Part model, mm, in its own coordinate system. A direction names the side the tool comes from. Round coordinates to 2 decimals unless told otherwise and drop trailing zeros. Order: outer loops, then holes, each group sorted by start corner. A loop starts at its lowest first (then second) coordinate and runs counter-clockwise, first axis right, second up. Notation, with made-up numbers: (36, 76) - (64, 76) arc R24 cw to (64, 92) - close; hole circle Ø6 at (11.25, -35). An arc over 180 degrees is marked (long way). Answer as a JSON object with one key per item and string values.
```python
from build123d import *

# Parameters (mm, degrees)
RESSALTO_EXTRUS_O1_DEPTH                             = 1000
CORTE_EXTRUS_O1_START                                = -1000
CORTE_EXTRUS_O1_DEPTH                                = 1000
CORTE_EXTRUS_O2_DEPTH                                = 1001.031261626
CORTE_EXTRUS_O3_DEPTH                                = 1001.031261626
CORTE_EXTRUS_O4_DEPTH                                = 1001.031261626
CORTE_EXTRUS_O5_DEPTH                                = 0.002166667
CORTE_EXTRUS_O6_DEPTH                                = 0.002166667
CORTE_EXTRUS_O7_DEPTH                                = 0.002166667
CORTE_EXTRUS_O8_DEPTH                                = 0.002166667
INCLINA_O1_ANGLE                                     = 45.1469538
ESBO_O10_W                                           = 0.450000001
ESBO_O10_H                                           = 1000
REBAIXO_PARA_PARAFUSO_DE_M_QUINA_DE_CABE_D           = 3.5
REBAIXO_PARA_PARAFUSO_DE_M_QUINA_DE_CABE_CBORE_D     = 6
REBAIXO_PARA_PARAFUSO_DE_M_QUINA_DE_CABE_CBORE_DEPTH = 3.50000002
CHANFRO1_SIZE                                        = 0.062563219
CHANFRO1_SIZE2                                       = 0.062205617
CHANFRO3_START                                       = -3.730761794
CHANFRO3_DEPTH                                       = 0.399013115
CHANFRO4_SIZE                                        = 0.4
FILETE1_R                                            = 0.130000023
SKETCH1_W                                            = 36.072768502
SKETCH1_H                                            = 858.120887339
SKETCH1_W_2                                          = 21.632087489
SKETCH1_H_2                                          = 62.411000867
CUT_EXTRUDE1_DEPTH                                   = 10


with BuildPart() as part:
    # Esboço1 → Ressalto-extrusão1 (new body)
    with BuildSketch(Plane.XZ):
        with BuildLine():
            Line((4.5, 5.4097155), (4.5, 6.01167813))
            Line((4.5, 6.01167813), (4.1, 6.50000002))
            Line((4.1, 6.50000002), (-4.1, 6.50000002))
            Line((-4.1, 6.50000002), (-4.5, 6.01167813))
            Line((-4.5, 6.01167813), (-4.5, 2e-08))
            Line((-4.5, 2e-08), (4.5, 2e-08))
            Line((4.5, 2e-08), (4.5, 3.50196265))
            ThreePointArc((4.5, 3.50196265), (4.477413879, 3.553810372), (4.43494978, 3.59116167))
            ThreePointArc((4.43494978, 3.59116167), (3.930462682, 4.43021964), (4.43494978, 5.26927761))
            ThreePointArc((4.43494978, 5.26927761), (4.490651601, 5.328761203), (4.5, 5.4097155))
        make_face()
    extrude(amount=-RESSALTO_EXTRUS_O1_DEPTH)

    # Esboço2 → Corte-extrusão1 (cut)
    with BuildSketch(Plane(origin=(0, 1000, 0), x_dir=(-1, 0, 0), z_dir=(0, 1, 0)).offset(CORTE_EXTRUS_O1_START)):
        with BuildLine():
            Line((-4.030498711, 4.00588336), (-3.673447948, 4.00588336))
            ThreePointArc((-3.673447948, 4.00588336), (-3.223447946, 4.455883362), (-3.673447948, 4.905883363))
            Line((-3.673447948, 4.905883363), (-3.953580008, 4.905883363))
            ThreePointArc((-3.953580008, 4.905883363), (-4.010719931, 4.899199784), (-4.065149208, 4.917830263))
            ThreePointArc((-4.065149208, 4.917830263), (-3.93114763, 4.466290066), (-4.030498711, 4.00588336))
        make_face()
    extrude(amount=CORTE_EXTRUS_O1_DEPTH, mode=Mode.SUBTRACT)

    # Esboço3 → Corte-extrusão2 (cut, through all)
    with BuildSketch(Plane(origin=(0, 1000, 0), x_dir=(-1, 0, 0), z_dir=(0, 1, 0))):
        with BuildLine():
            Line((4.5, 4.03150278), (4.5, 4.88017535))
            Line((4.5, 4.88017535), (3.66946318, 4.88017535))
            ThreePointArc((3.66946318, 4.88017535), (3.969667593, 4.455839065), (3.66946318, 4.03150278))
            Line((3.66946318, 4.03150278), (4.5, 4.03150278))
        make_face()
    extrude(amount=-CORTE_EXTRUS_O2_DEPTH, mode=Mode.SUBTRACT)

    # Esboço4 → Corte-extrusão3 (cut, through all)
    with BuildSketch(Plane(origin=(0, 1000, 0), x_dir=(-1, 0, 0), z_dir=(0, 1, 0))):
        with BuildLine():
            Line((4.026513974, 4.88017535), (4.5, 4.88017535))
            Line((4.5, 4.88017535), (4.5, 5.328056964))
            ThreePointArc((4.5, 5.328056964), (4.223646078, 5.145991535), (4.026513974, 4.88017535))
        make_face()
    extrude(amount=-CORTE_EXTRUS_O3_DEPTH, mode=Mode.SUBTRACT)

    # Esboço5 → Corte-extrusão4 (cut, through all)
    with BuildSketch(Plane(origin=(0, 1000, 0), x_dir=(-1, 0, 0), z_dir=(0, 1, 0))):
        with BuildLine():
            Line((4.5, 3.583620931), (4.5, 4.03150278))
            Line((4.5, 4.03150278), (4.026513856, 4.03150278))
            ThreePointArc((4.026513856, 4.03150278), (4.223645982, 3.76568645), (4.5, 3.583620931))
        make_face()
    extrude(amount=-CORTE_EXTRUS_O4_DEPTH, mode=Mode.SUBTRACT)

    # Esboço6 → Corte-extrusão5 (cut)
    with BuildSketch(Plane(origin=(0, 1000, 0), x_dir=(-1, 0, 0), z_dir=(0, 1, 0))):
        Polygon((0.891369267, 3.403698133), (0.714701433, 3.168235633), (0.2187042, 2.61105), (1.0945792, 2.61105), (1.0945792, 2.695983333), (0.398689633, 2.695983333), (0.794326433, 3.149466667), (0.9743123, 3.3891), (1.067110588, 3.573407857), (0.95413722, 3.802321701), (0.7876908, 3.88505), (0.54301, 3.88505), (0.375434678, 3.803592619), (0.295011167, 3.6384023), (0.295011167, 3.562), (0.3812718, 3.562), (0.3812718, 3.631766667), (0.437672733, 3.743620833), (0.549645633, 3.800116667), (0.7802262, 3.800116667), (0.893028067, 3.743810633), (0.976240026, 3.576039029), align=None)
    extrude(amount=-CORTE_EXTRUS_O5_DEPTH, mode=Mode.SUBTRACT)

    # Esboço7 → Corte-extrusão6 (cut)
    with BuildSketch(Plane.XZ):
        Polygon((-0.214632167, 3.88505), (-0.953983333, 3.88505), (-0.953983333, 2.61105), (-0.214632167, 2.61105), (-0.214632167, 2.695983333), (-0.86905, 2.695983333), (-0.86905, 3.205583333), (-0.5123963, 3.205583333), (-0.5123963, 3.290516667), (-0.86905, 3.290516667), (-0.86905, 3.800116667), (-0.214632167, 3.800116667), align=None)
    extrude(amount=-CORTE_EXTRUS_O6_DEPTH, mode=Mode.SUBTRACT)

    # Esboço8 → Corte-extrusão7 (cut)
    with BuildSketch(Plane(origin=(0, 1000, 0), x_dir=(-1, 0, 0), z_dir=(0, 1, 0))):
        Polygon((-0.214632167, 3.88505), (-0.953983333, 3.88505), (-0.953983333, 2.61105), (-0.214632167, 2.61105), (-0.214632167, 2.695983333), (-0.86905, 2.695983333), (-0.86905, 3.205583333), (-0.5123963, 3.205583333), (-0.5123963, 3.290516667), (-0.86905, 3.290516667), (-0.86905, 3.800116667), (-0.214632167, 3.800116667), align=None)
    extrude(amount=-CORTE_EXTRUS_O7_DEPTH, mode=Mode.SUBTRACT)

    # Esboço9 → Corte-extrusão8 (cut)
    with BuildSketch(Plane.XZ):
        Polygon((0.510057167, 3.620830633), (0.6071, 3.718655633), (0.6071, 2.609403333), (0.692033333, 2.609403333), (0.692033333, 3.883403333), (0.6741176, 3.883403333), (0.6741176, 3.795069794), (0.3690544, 3.640736667), (0.3690544, 3.551253333), align=None)
    extrude(amount=-CORTE_EXTRUS_O8_DEPTH, mode=Mode.SUBTRACT)

    # Inclinação1
    inclina_o1_faces = [part.faces().sort_by_distance(p)[0] for p in [
        (0.6741176, 0.001083333, 3.839236564),
    ]]
    draft(inclina_o1_faces, Plane(origin=(0.692033333, 0.002166667, 3.883403333), x_dir=(-1, 0, 0), z_dir=(0, 0, -1)), INCLINA_O1_ANGLE)

    # Esboço10 → Corte-Revolução1 (revolve, cut)
    with BuildSketch(Plane.XY.offset(4.455839065)):
        with Locations((-3.294667591, 500)):
            Rectangle(ESBO_O10_W, ESBO_O10_H)
    revolve(axis=Axis((-3.519667591, 1000, 4.455839065), (0, -1, 0)), mode=Mode.SUBTRACT)

    # Rebaixo para parafuso de máquina de cabeça sextavada de M31 (through all)
    with Locations(Plane.XY.offset(6.50000002)):
        with Locations((0, 990), (0, 970), (0, 950), (0, 930), (0, 910), (0, 890), (0, 870), (0, 850), (0, 830), (0, 810), (0, 790), (0, 770), (0, 750), (0, 730), (0, 710), (0, 690), (0, 670), (0, 650), (0, 630), (0, 610), (0, 590), (0, 570), (0, 550), (0, 530), (0, 510), (0, 490), (0, 470), (0, 450), (0, 430), (0, 410), (0, 390), (0, 370), (0, 350), (0, 330), (0, 310), (0, 290), (0, 270), (0, 250), (0, 230), (0, 210), (0, 190), (0, 170), (0, 150), (0, 130), (0, 110), (0, 90), (0, 70), (0, 50), (0, 30), (0, 10)):
            CounterBoreHole(REBAIXO_PARA_PARAFUSO_DE_M_QUINA_DE_CABE_D / 2, REBAIXO_PARA_PARAFUSO_DE_M_QUINA_DE_CABE_CBORE_D / 2, REBAIXO_PARA_PARAFUSO_DE_M_QUINA_DE_CABE_CBORE_DEPTH)

    # Chanfro1
    chanfro1_edges = [part.edges().sort_by_distance(p)[0] for p in [
        (-0.976240026, 999.998916667, 3.576039029),
    ]]
    chanfro1_side = [part.faces().sort_by_distance(p)[0] for p in [
        (-0.933804646, 999.998916667, 3.489868581),
    ]]
    chamfer(chanfro1_edges, length=CHANFRO1_SIZE, length2=CHANFRO1_SIZE2, reference=chanfro1_side[0])

    # Chanfro3: read off the stored shape, not the designer's step
    # Chanfro3 outline → Chanfro3 (add)
    with BuildSketch(Plane(origin=(0, 0, 0), x_dir=(0.8991051825477068, 0, 0.43773264753254887), z_dir=(0.4377326475325489, 0, -0.8991051825477069)).offset(CHANFRO3_START)):
        Polygon((1.327401403, -999.997833333), (1.31122788, -999.997833333), (1.311999664, -1000), (1.327401403, -1000), align=None)
    extrude(amount=CHANFRO3_DEPTH)

    # Chanfro4
    chanfro4_edges = [part.edges().sort_by_distance(p)[0] for p in [
        (4.5, 500, 2e-08),
        (-4.5, 500, 2e-08),
    ]]
    chamfer(chanfro4_edges, length=CHANFRO4_SIZE)

    # Filete1
    filete1_edges = [part.edges().sort_by_distance(p)[0] for p in [
        (4.030498711, 500, 4.00588336),
        (-4.026513974, 500, 4.88017535),
        (-4.5, 500, 5.328056964),
        (-4.5, 500, 3.583620931),
        (-4.026513856, 500, 4.03150278),
    ]]
    fillet(filete1_edges, radius=FILETE1_R)

    # Sketch1 → Cut-Extrude1 (cut)
    with BuildSketch(Plane(origin=(0, 0, 0), x_dir=(-1, 0, 0), z_dir=(0, 0, -1))):
        with Locations((-9.39117436, 589.29269367)):
            Rectangle(SKETCH1_W, SKETCH1_H)
        with Locations((0.25600221, -13.052857141)):
            Rectangle(SKETCH1_W_2, SKETCH1_H_2)
    extrude(amount=-CUT_EXTRUDE1_DEPTH, mode=Mode.SUBTRACT)


solid = part.part
```
Item 1: Tool access for faces 4 (the cylindrical face through (-0.81, 28.45, 1.48)), 5 (the flat face through (0, 128, 3)): list every direction of +Z, -Z, +X, -X, +Y, -Y with a clear straight run to the whole face (end or side of a thin tool).
Taken from the geometry:
{"face 4": "+Z, -Z", "face 5": "+Z"}
Item 2: Probe L1, parallel to Z at x = -4, y = 149.5; L2, parallel to X at y = 90, z = 1.5; L3, parallel to X at y = 89, z = 2.25. List the from-to ranges inside material, lowest first. Write a range as from..to.
Taken from the geometry:
{"L1": "0..4.02, 4.89..6.5", "L2": "-4.5..-1.75, 1.75..4.5", "L3": "-4.5..-1.44, 1.44..4.5"}
Item 3: Drop flat-ended pins along their axis: P1, Ø1.8, axis at x = -1.5, y = 130, coming from the +Z side; P2, Ø0.5, axis at y = 75, z = 6, coming from the +X side; P3, Ø3, axis at x = 0, y = 110, coming from the +Z side. Give the stop position or say it passes through.
Taken from the geometry:
{"P1": "z = 3", "P2": "x = 4.5", "P3": "through"}
Item 4: Two-plate mould, pull along Y, no slides. Class faces 1 (the flat face through (4.5, 88, 2)), 2 (the flat face through (2, 110, 3)), 3 (the flat face through (0, 160.232, 3)): pulls with the +Y half, pulls with the -Y half, needs draft (parallel to the pull), parting line crosses it, or undercut.
Taken from the geometry:
{"face 1": "needs draft", "face 2": "undercut", "face 3": "pulls with the +Y half"}
Item 5: Cut at A-A (y = 125). Write the cut outline in (x, z), plus the area to 3 significant figures.
Taken from the geometry:
{"outline": "(-4.5, 0.4) - (-4.1, 0) - (4.1, 0) - (4.5, 0.4) - (4.5, 3.5) arc R0.13 ccw to (4.43, 3.59) arc R0.95 cw to (4.07, 3.94) arc R0.13 ccw to (3.95, 4.01) - (3.67, 4.01) arc R0.45 cw to (3.67, 4.91) - (3.95, 4.91) arc R0.13 ccw to (4.07, 4.92) arc R0.95 cw to (4.43, 5.27) arc R0.13 ccw to (4.5, 5.41) - (4.5, 6.01) - (4.1, 6.5) - (-4.1, 6.5) - (-4.5, 6.01) - (-4.5, 5.41) arc R0.13 ccw to (-4.43, 5.29) arc R0.95 cw to (-4.06, 4.94) arc R0.13 ccw to (-3.95, 4.88) - (-3.67, 4.88) arc R0.45 cw (long way) to (-3.67, 4.03) - (-3.95, 4.03) arc R0.13 ccw to (-4.06, 3.97) arc R0.95 cw to (-4.43, 3.62) arc R0.13 ccw to (-4.5, 3.5) - close", "area": "55.4 mm2"}
